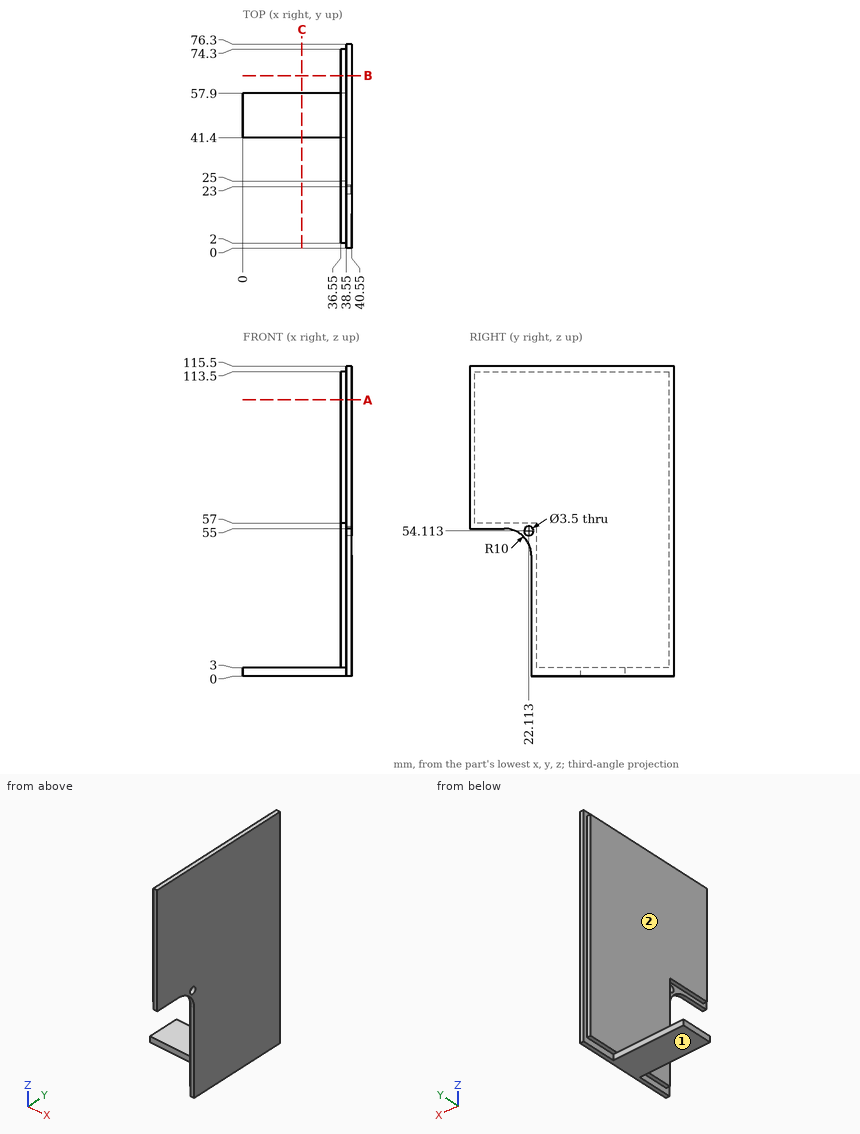
Check sheet for the drawn part. Datum: minimum x, y, z corner. Units: mm. A direction names the side the tool comes from. Give positions to 0.01 mm unless a question says otherwise; leave off trailing zeros. Write each loop counter-clockwise with the first axis right and the second up, starting at its lowest first coordinate (ties: lowest second). Pieces come first, ordered by that corner, then holes.
(1) Gauge pin test, flat ends, axial feed: pin 1 (2 mm diameter, centred on x = 37.5, y = 9.5, fed in from -Z); pin 2 (1 mm diameter, centred on x = 38, y = 68.5, fed in from -Z); pin 3 (1 mm diameter, centred on x = 39.5, y = 7.5, fed in from -Z); pin 4 (8 mm diameter, centred on x = 32, y = 17.5, fed in from +Z). Record the tip position at first contact, or that the pin passes through.
(2) Access from +Z, -Z, +X, -X, +Y, -Y to the whole of each face (thin tool, end or side, straight path). Record for the marked faces 1 and 2.
(3) Cross-section at A-A (z = 103). Enter the section's corners in (x, y), plus the area to 3 significant figures.
(4) Cross-section at C-C (x = 22). Enter the section's corners in (y, z), plus the area to 3 significant figures.
(5) Material ranges on line 1 (X direction, y = 46.5, z = 10); line 2 (Z direction, x = 37, y = 40); line 3 (Z direction, x = 34, y = 52), recorded low to high.
(6) Cross-section at B-B (y = 64.5). Enter the section's corners in (x, z).
Worked out:
1. pin 1: stops at z = 57
1. pin 2: stops at z = 3
1. pin 3: stops at z = 55
1. pin 4: passes through
2. face 1: -Z, +X, -X, +Y, -Y
2. face 2: +Z, -X, +Y, -Y
3. outline: (36.55, 2) - (38.55, 2) - (38.55, 0) - (40.55, 0) - (40.55, 76.3) - (38.55, 76.3) - (38.55, 74.3) - (36.55, 74.3) - close
3. area: 297 mm2
4. outline: (41.4, 0) - (57.9, 0) - (57.9, 3) - (41.4, 3) - close
4. area: 49.5 mm2
5. line 1: x = 36.55 to 40.55
5. line 2: z = 3 to 113.5
5. line 3: z = 0 to 3
6. outline: (36.55, 3) - (38.55, 3) - (38.55, 0) - (40.55, 0) - (40.55, 115.5) - (38.55, 115.5) - (38.55, 113.5) - (36.55, 113.5) - close
